from build123d import *

# Parameters (mm, degrees)
SKETCH_1_R          = 21
EXTRUDE_1_DEPTH     = 20
EXTRUDE_2_DEPTH     = 20
SKETCH_6_R          = 35
CUT_EXTRUDE_4_DEPTH = 13
SKETCH_4_R          = 2.5
SKETCH_4_R_2        = 12
CUT_EXTRUDE_3_DEPTH = 21
SKETCH_7_W          = 45
SKETCH_7_H          = 45
CUT_EXTRUDE_5_DEPTH = 15
SKETCH_2_R          = 6
CUT_EXTRUDE_1_DEPTH = 54
SKETCH_3_R          = 3.1
CUT_EXTRUDE_2_DEPTH = 17.320508076
SKETCH_8_R          = 6
CUT_EXTRUDE_6_DEPTH = 61
SKETCH_9_R          = 3.1
CUT_EXTRUDE_7_DEPTH = 15.320508076
FILLET_1_R          = 8
SKETCH_10_W         = 12
SKETCH_10_H         = 22
SKETCH_10_W_2       = 35
SKETCH_10_H_2       = 12
CUT_EXTRUDE_8_DEPTH = 21
FILLET_2_R          = 2


with BuildPart() as part:
    # Эскиз1 → Бобышка-Вытянуть1 (new body)
    with BuildSketch(Plane(origin=(0, 0, 0), x_dir=(1, 0, 0), z_dir=(0, 1, 0))):
        with BuildLine():
            Line((-11, 43.634848459), (-11, 95))
            Line((-11, 95), (11, 95))
            Line((11, 95), (11, 43.634848459))
            ThreePointArc((11, 43.634848459), (31.819805153, 31.819805153), (43.634848459, 11))
            Line((43.634848459, 11), (105, 11))
            Line((105, 11), (105, -11))
            Line((105, -11), (43.634848459, -11))
            ThreePointArc((43.634848459, -11), (31.819805153, -31.819805153), (11, -43.634848459))
            Line((11, -43.634848459), (11, -95))
            Line((11, -95), (-11, -95))
            Line((-11, -95), (-11, -43.634848459))
            ThreePointArc((-11, -43.634848459), (-31.819805153, -31.819805153), (-43.634848459, -11))
            Line((-43.634848459, -11), (-105, -11))
            Line((-105, -11), (-105, 11))
            Line((-105, 11), (-43.634848459, 11))
            ThreePointArc((-43.634848459, 11), (-31.819805153, 31.819805153), (-11, 43.634848459))
        make_face()
        Circle(SKETCH_1_R, mode=Mode.SUBTRACT)
    extrude(amount=EXTRUDE_1_DEPTH)

    # Эскиз5 → Бобышка-Вытянуть2 (add, through all)
    with BuildSketch(Plane(origin=(0, 20, 0), x_dir=(1, 0, 0), z_dir=(0, 1, 0))):
        with BuildLine():
            Line((-35.619517122, 27.5), (-90.619517122, 27.5))
            Line((-90.619517122, 27.5), (-90.619517122, 11))
            Line((-90.619517122, 11), (-43.634848459, 11))
            ThreePointArc((-43.634848459, 11), (-40.476859017, 19.662753726), (-35.619517122, 27.5))
        make_face()
        with BuildLine():
            Line((-35.619517122, -27.5), (-90.619517122, -27.5))
            Line((-90.619517122, -27.5), (-90.619517122, -11))
            Line((-90.619517122, -11), (-43.634848459, -11))
            ThreePointArc((-43.634848459, -11), (-40.476859017, -19.662753726), (-35.619517122, -27.5))
        make_face()
    extrude(amount=-EXTRUDE_2_DEPTH)

    # Эскиз6 → Вырез-Вытянуть4 (cut)
    with BuildSketch(Plane(origin=(0, 20, 0), x_dir=(1, 0, 0), z_dir=(0, 1, 0))):
        Circle(SKETCH_6_R)
    extrude(amount=-CUT_EXTRUDE_4_DEPTH, mode=Mode.SUBTRACT)

    # Эскиз4 → Вырез-Вытянуть3 (cut, through all)
    with BuildSketch(Plane(origin=(0, 20, 0), x_dir=(1, 0, 0), z_dir=(0, 1, 0))):
        with Locations((-47, 15.5)):
            Circle(SKETCH_4_R)
        with Locations((-78, 15.5)):
            Circle(SKETCH_4_R)
        with Locations((-78, -15.5)):
            Circle(SKETCH_4_R)
        with Locations((-47, -15.5)):
            Circle(SKETCH_4_R)
        with Locations((-62.5, 0)):
            Circle(SKETCH_4_R_2)
    extrude(amount=-CUT_EXTRUDE_3_DEPTH, mode=Mode.SUBTRACT)

    # Эскиз7 → Вырез-Вытянуть5 (cut)
    with BuildSketch(Plane.XZ):
        with Locations((-62.5, 0)):
            Rectangle(SKETCH_7_W, SKETCH_7_H)
    extrude(amount=-CUT_EXTRUDE_5_DEPTH, mode=Mode.SUBTRACT)

    # Эскиз2 → Вырез-Вытянуть1 (cut)
    with BuildSketch(Plane(origin=(0, 19.763139721, 11.410254038), x_dir=(1, 0, 0), z_dir=(0, 0.866025404, 0.5))):
        with Locations((0, 77.27241336)):
            Circle(SKETCH_2_R)
    cut_extrude_1 = extrude(amount=-CUT_EXTRUDE_1_DEPTH, mode=Mode.SUBTRACT)

    # Эскиз3 → Вырез-Вытянуть2 (cut, through all)
    with BuildSketch(Plane(origin=(0, -27.002232084, -15.589745962), x_dir=(1, 0, 0), z_dir=(0, 0.866025404, 0.5))):
        with Locations((0, 77.27241336)):
            Circle(SKETCH_3_R)
    cut_extrude_2 = extrude(amount=-CUT_EXTRUDE_2_DEPTH, mode=Mode.SUBTRACT)

    # Эскиз8 → Вырез-Вытянуть6 (cut)
    with BuildSketch(Plane(origin=(11.410254038, 19.763139721, 0), x_dir=(0, 0, -1), z_dir=(0.5, 0.866025404, 0))):
        with Locations((0, 87.432667397)):
            Circle(SKETCH_8_R)
    cut_extrude_6 = extrude(amount=-CUT_EXTRUDE_6_DEPTH, mode=Mode.SUBTRACT)

    # Эскиз9 → Вырез-Вытянуть7 (cut, through all)
    with BuildSketch(Plane(origin=(-19.089745962, -33.06440991, 0), x_dir=(0.866025404, -0.5, 0), z_dir=(0.5, 0.866025404, 0))):
        with Locations((-87.432667397, 0)):
            Circle(SKETCH_9_R)
    cut_extrude_7 = extrude(amount=-CUT_EXTRUDE_7_DEPTH, mode=Mode.SUBTRACT)

    # Скругление1
    fillet_1_edges = [part.edges().sort_by_distance(p)[0] for p in [
        (-11, 10, -95),
        (11, 10, -95),
        (105, 10, -11),
        (105, 10, 11),
        (11, 10, 95),
        (-11, 10, 95),
        (-105, 10, 11),
        (-105, 10, -11),
        (-90.619517122, 10, -27.5),
        (-90.619517122, 10, 27.5),
    ]]
    fillet(fillet_1_edges, radius=FILLET_1_R)

    # Зеркальное отражение1: Вырез-Вытянуть1, Вырез-Вытянуть2 across plane
    add(cut_extrude_1.mirror(Plane.XY), mode=Mode.SUBTRACT)
    add(cut_extrude_2.mirror(Plane.XY), mode=Mode.SUBTRACT)

    # Зеркальное отражение2: Вырез-Вытянуть6, Вырез-Вытянуть7 across plane
    add(cut_extrude_6.mirror(Plane(origin=(0, 0, 0), x_dir=(0, 0, 1), z_dir=(1, 0, 0))), mode=Mode.SUBTRACT)
    add(cut_extrude_7.mirror(Plane(origin=(0, 0, 0), x_dir=(0, 0, 1), z_dir=(1, 0, 0))), mode=Mode.SUBTRACT)

    # Эскиз10 → Вырез-Вытянуть8 (cut, through all)
    with BuildSketch(Plane(origin=(0, 20, 0), x_dir=(1, 0, 0), z_dir=(0, 1, 0))):
        with Locations((0, 56)):
            Rectangle(SKETCH_10_W, SKETCH_10_H)
        with Locations((62.5, 0)):
            Rectangle(SKETCH_10_W_2, SKETCH_10_H_2)
        with Locations((0, -56)):
            Rectangle(SKETCH_10_W, SKETCH_10_H)
    extrude(amount=-CUT_EXTRUDE_8_DEPTH, mode=Mode.SUBTRACT)

    # Скругление2
    fillet_2_edges = [part.edges().sort_by_distance(p)[0] for p in [
        (6, 10, -67),
        (6, 10, -45),
        (-6, 10, -45),
        (-6, 10, -67),
        (80, 10, -6),
        (80, 10, 6),
        (45, 10, 6),
        (45, 10, -6),
        (-6, 10, 67),
        (-6, 10, 45),
        (6, 10, 45),
        (6, 10, 67),
    ]]
    fillet(fillet_2_edges, radius=FILLET_2_R)


solid = part.part
The listing builds one solid part. Answer for the finished solid, in the listing's coordinates (mm). A direction names the side the tool comes from. Round coordinates to 2 decimals unless told otherwise and drop trailing zeros. Order: outer loops, then holes, each group sorted by start corner. A loop starts at its lowest first (then second) coordinate and runs counter-clockwise, first axis right, second up. Notation, with made-up numbers: (88.5, 14) -> (143.5, 14) arc R13 cw to (143.5, 36) -> close; hole circle Ø2 at (41.5, 74). An arc over 180 degrees is marked (long way). One line per item, written item: value.
Item 1: Find section A-A, the plane x = 53.5. Give the vertices of the cut face in (y, z), then the cut area to 3 significant figures.
Taken from the geometry:
outline: (0, -11) -> (20, -11) -> (20, -6) -> (0, -6) -> close; (0, 6) -> (20, 6) -> (20, 11) -> (0, 11) -> close
area: 200 mm2
Item 2: Find section D-D, the plane z = 15.5. Give the vertices of the cut face in (x, y), then the cut area to 3 significant figures.
Taken from the geometry:
outline: (-90.62, 0) -> (-85, 0) -> (-85, 15) -> (-80.5, 15) -> (-80.5, 20) -> (-90.62, 20) -> close; (-75.5, 15) -> (-49.5, 15) -> (-49.5, 20) -> (-75.5, 20) -> close; (-44.5, 15) -> (-40, 15) -> (-40, 0) -> (-14.17, 0) -> (-14.17, 7) -> (-31.38, 7) -> (-31.38, 20) -> (-44.5, 20) -> close; (14.17, 0) -> (42.25, 0) -> (42.25, 20) -> (31.38, 20) -> (31.38, 7) -> (14.17, 7) -> close
area: 918 mm2
Item 3: For faces 1 (the flat face through (71, 10, 11)), 2 (the flat face through (-6, 10, -56)), 3 (the flat face through (-11, 10, 66)), determine the directions among +Z, -Z, +X, -X, +Y, -Y from which every point of the face is accessible in a straight line to the end or side of a thin tool.
Taken from the geometry:
face 1: +Z, +X, +Y, -Y
face 2: +Y, -Y
face 3: +Z, -X, +Y, -Y
Item 4: Find section C-C, the plane z = -57.5. Give the vertices of the cut face in (x, y).
Taken from the geometry:
outline: (-11, 0) -> (-6, 0) -> (-6, 20) -> (-11, 20) -> close; (6, 0) -> (11, 0) -> (11, 20) -> (6, 20) -> close
Item 5: Given P1, Ø19, axis at x = -62.5, z = 0, coming from the +Y side; P2, Ø6, axis at y = 8.5, z = 16, coming from the -X side; P3, Ø7.5, axis at x = -51.5, y = 10.5, coming from the -Z side; P4, Ø1.5, axis at y = 18, z = 61.5, coming from the -X side, each flat-ended and moving along its own axis, determine where each tip first touches the part or whether it passes through.
Taken from the geometry:
P1: passes through
P2: stops at x = -90.62
P3: stops at z = -27.5
P4: stops at x = -11
Item 6: For a pull along X with two mould halves and no side action, classify faces 4 (the flat face through (-90.62, 10, -15)), 5 (the flat face through (-94, 10, -11)), 6 (the flat face through (62, 10, -6)) as released by +X, released by -X, zero draft, split by the parting line, or undercut.
Taken from the geometry:
face 4: released by -X
face 5: zero draft
face 6: undercut
Item 7: Straight lines are drawn through the part: L1, parallel to Z at x = -78, y = 16.9; L2, parallel to Z at x = 62.5, y = 18.75; L3, parallel to Z at x = -62.5, y = 18.15. For each, find the intervals that lie inside material, in ascending order.
Taken from the geometry:
L1: z = -27.5 to -18, -13 to 13, 18 to 27.5
L2: z = -11 to -6, 6 to 11
L3: z = -27.5 to -12, 12 to 27.5
Item 8: Find section B-B, the plane x = -47. Give the vertices of the cut face in (y, z), then the cut area to 3 significant figures.
Taken from the geometry:
outline: (0, -27.5) -> (20, -27.5) -> (20, -18) -> (15, -18) -> (15, -22.5) -> (0, -22.5) -> close; (0, 22.5) -> (15, 22.5) -> (15, 18) -> (20, 18) -> (20, 27.5) -> (0, 27.5) -> close; (15, -13) -> (20, -13) -> (20, 13) -> (15, 13) -> close
area: 375 mm2
